from build123d import *

# Parameters (mm, degrees)
SKETCH1_R           = 57.5
SKETCH1_R_2         = 1.6
BOSS_EXTRUDE1_DEPTH = 10.6
FILLET1_R           = 2.5


with BuildPart() as part:
    # Sketch1 → Boss-Extrude1 (new body)
    with BuildSketch(Plane(origin=(0, 0, 0), x_dir=(1, 0, 0), z_dir=(0, 1, 0))):
        with Locations(Location((0, 0, 0), (0, 0, 270))):
            Circle(SKETCH1_R)
        with Locations(Location((-27, -46.765371804, 0), (0, 0, 270))):
            Circle(SKETCH1_R_2, mode=Mode.SUBTRACT)
        with Locations(Location((-46.765371804, -27, 0), (0, 0, 270))):
            Circle(SKETCH1_R_2, mode=Mode.SUBTRACT)
        with Locations(Location((-54, 0, 0), (0, 0, 270))):
            Circle(SKETCH1_R_2, mode=Mode.SUBTRACT)
        with Locations(Location((0, -54, 0), (0, 0, 270))):
            Circle(SKETCH1_R_2, mode=Mode.SUBTRACT)
        with Locations(Location((27, -46.765371804, 0), (0, 0, 270))):
            Circle(SKETCH1_R_2, mode=Mode.SUBTRACT)
        with BuildLine():
            ThreePointArc((43.742247125, 10.564838686), (44.135337618, 8.779064491), (44.455555556, 6.978795043))
            ThreePointArc((44.455555556, 6.978795043), (49.753361384, 5.138633627), (52, 0))
            ThreePointArc((52, 0), (49.753361384, -5.138633627), (44.455555556, -6.978795043))
            ThreePointArc((44.455555556, -6.978795043), (44.135337618, -8.779064491), (43.742247125, -10.564838686))
            ThreePointArc((43.742247125, -10.564838686), (47.23910353, -13.108193036), (48.574578963, -17.220754456))
            ThreePointArc((48.574578963, -17.220754456), (45.234108152, -23.187985482), (38.400908644, -23.459970489))
            ThreePointArc((38.400908644, -23.459970489), (37.416132554, -25.000660486), (36.369578094, -26.500071496))
            ThreePointArc((36.369578094, -26.500071496), (38.177808401, -28.89135937), (38.819805153, -31.819805153))
            ThreePointArc((38.819805153, -31.819805153), (34.244868492, -38.386316236), (26.500071496, -36.369578094))
            ThreePointArc((26.500071496, -36.369578094), (25.000660486, -37.416132554), (23.459970489, -38.400908644))
            ThreePointArc((23.459970489, -38.400908644), (24.027901885, -39.942787345), (24.220754456, -41.574578963))
            ThreePointArc((24.220754456, -41.574578963), (18.318158122, -48.488022764), (10.564838686, -43.742247125))
            ThreePointArc((10.564838686, -43.742247125), (8.779064491, -44.135337618), (6.978795043, -44.455555556))
            ThreePointArc((6.978795043, -44.455555556), (6.994696752, -44.727571384), (7, -45))
            ThreePointArc((7, -45), (-0.272428616, -51.994696752), (-6.978795043, -44.455555556))
            ThreePointArc((-6.978795043, -44.455555556), (-8.779064491, -44.135337618), (-10.564838686, -43.742247125))
            ThreePointArc((-10.564838686, -43.742247125), (-19.899538483, -48.041735691), (-23.459970489, -38.400908644))
            ThreePointArc((-23.459970489, -38.400908644), (-25.000660486, -37.416132554), (-26.500071496, -36.369578094))
            ThreePointArc((-26.500071496, -36.369578094), (-36.769552622, -36.769552622), (-36.369578094, -26.500071496))
            ThreePointArc((-36.369578094, -26.500071496), (-37.416132554, -25.000660486), (-38.400908644, -23.459970489))
            ThreePointArc((-38.400908644, -23.459970489), (-48.041735691, -19.899538483), (-43.742247125, -10.564838686))
            ThreePointArc((-43.742247125, -10.564838686), (-44.135337618, -8.779064491), (-44.455555556, -6.978795043))
            ThreePointArc((-44.455555556, -6.978795043), (-52, 0), (-44.455555556, 6.978795043))
            ThreePointArc((-44.455555556, 6.978795043), (-44.135337618, 8.779064491), (-43.742247125, 10.564838686))
            ThreePointArc((-43.742247125, 10.564838686), (-48.041735691, 19.899538483), (-38.400908644, 23.459970489))
            ThreePointArc((-38.400908644, 23.459970489), (-37.416132554, 25.000660486), (-36.369578094, 26.500071496))
            ThreePointArc((-36.369578094, 26.500071496), (-36.769552622, 36.769552622), (-26.500071496, 36.369578094))
            ThreePointArc((-26.500071496, 36.369578094), (-25.000660486, 37.416132554), (-23.459970489, 38.400908644))
            ThreePointArc((-23.459970489, 38.400908644), (-19.899538483, 48.041735691), (-10.564838686, 43.742247125))
            ThreePointArc((-10.564838686, 43.742247125), (-8.779064491, 44.135337618), (-6.978795043, 44.455555556))
            ThreePointArc((-6.978795043, 44.455555556), (-0.272428616, 51.994696752), (7, 45))
            ThreePointArc((7, 45), (6.994696752, 44.727571384), (6.978795043, 44.455555556))
            ThreePointArc((6.978795043, 44.455555556), (8.779064491, 44.135337618), (10.564838686, 43.742247125))
            ThreePointArc((10.564838686, 43.742247125), (18.318158122, 48.488022764), (24.220754456, 41.574578963))
            ThreePointArc((24.220754456, 41.574578963), (24.027901885, 39.942787345), (23.459970489, 38.400908644))
            ThreePointArc((23.459970489, 38.400908644), (25.000660486, 37.416132554), (26.500071496, 36.369578094))
            ThreePointArc((26.500071496, 36.369578094), (34.244868492, 38.386316236), (38.819805153, 31.819805153))
            ThreePointArc((38.819805153, 31.819805153), (38.177808401, 28.89135937), (36.369578094, 26.500071496))
            ThreePointArc((36.369578094, 26.500071496), (37.416132554, 25.000660486), (38.400908644, 23.459970489))
            ThreePointArc((38.400908644, 23.459970489), (45.234108152, 23.187985482), (48.574578963, 17.220754456))
            ThreePointArc((48.574578963, 17.220754456), (47.23910353, 13.108193036), (43.742247125, 10.564838686))
        make_face(mode=Mode.SUBTRACT)
        with Locations(Location((46.765371804, -27, 0), (0, 0, 270))):
            Circle(SKETCH1_R_2, mode=Mode.SUBTRACT)
        with Locations(Location((-46.765371804, 27, 0), (0, 0, 270))):
            Circle(SKETCH1_R_2, mode=Mode.SUBTRACT)
        with Locations(Location((-27, 46.765371804, 0), (0, 0, 270))):
            Circle(SKETCH1_R_2, mode=Mode.SUBTRACT)
        with Locations(Location((54, 0, 0), (0, 0, 270))):
            Circle(SKETCH1_R_2, mode=Mode.SUBTRACT)
        with Locations(Location((46.765371804, 27, 0), (0, 0, 270))):
            Circle(SKETCH1_R_2, mode=Mode.SUBTRACT)
        with Locations(Location((0, 54, 0), (0, 0, 270))):
            Circle(SKETCH1_R_2, mode=Mode.SUBTRACT)
        with Locations(Location((27, 46.765371804, 0), (0, 0, 270))):
            Circle(SKETCH1_R_2, mode=Mode.SUBTRACT)
    extrude(amount=BOSS_EXTRUDE1_DEPTH)

    # Fillet1
    # the kernel refuses this fillet: 2.5 mm, written as the material it takes off along each edge
    with BuildSketch(Plane(origin=(43.742247125, -4.820377086, -10.564838686), x_dir=(0.21389520927514544, 0, 0.9768566115091517), z_dir=(0, 1, 0)), Plane(origin=(44.455555556, -4.820377086, 6.978795043), x_dir=(-0.17621343506931061, 0, 0.9843519824234996), z_dir=(0, 1, 0)), Plane(origin=(38.400908644, -4.820377086, 23.459970489), x_dir=(-0.5394951813032318, 0, 0.841988687186825), z_dir=(0, 1, 0)), Plane(origin=(26.500071496, -4.820377086, 36.369578094), x_dir=(-0.8206436767197667, 0, 0.5714402469723874), z_dir=(0, 1, 0)), Plane(origin=(10.564838686, -4.820377086, 43.742247125), x_dir=(-0.9768566115091482, 0, 0.21389520927516179), z_dir=(0, 1, 0)), Plane(origin=(-6.978795043, -4.820377086, 44.455555556), x_dir=(-0.9843519824235082, 0, -0.1762134350692629), z_dir=(0, 1, 0)), Plane(origin=(-23.459970489, -4.820377086, 38.400908644), x_dir=(-0.8419886871868016, 0, -0.5394951813032682), z_dir=(0, 1, 0)), Plane(origin=(-36.369578094, -4.820377086, 26.500071496), x_dir=(-0.5714402469723492, 0, -0.8206436767197933), z_dir=(0, 1, 0)), Plane(origin=(23.459970489, -4.820377086, -38.400908644), x_dir=(0.8419886871867822, 0, 0.5394951813032985), z_dir=(0, 1, 0)), Plane(origin=(6.978795043, -4.820377086, -44.455555556), x_dir=(0.9843519824234905, 0, 0.1762134350693622), z_dir=(0, 1, 0)), Plane(origin=(-10.564838686, -4.820377086, -43.742247125), x_dir=(0.9768566115091611, 0, -0.21389520927510192), z_dir=(0, 1, 0)), Plane(origin=(-26.500071496, -4.820377086, -36.369578094), x_dir=(0.8206436767197971, 0, -0.5714402469723435), z_dir=(0, 1, 0)), Plane(origin=(-38.400908644, -4.820377086, -23.459970489), x_dir=(0.5394951813033058, 0, -0.8419886871867777), z_dir=(0, 1, 0)), Plane(origin=(-44.455555556, -4.820377086, -6.978795043), x_dir=(0.17621343506938397, 0, -0.9843519824234865), z_dir=(0, 1, 0)), Plane(origin=(-43.742247125, -4.820377086, 10.564838686), x_dir=(-0.21389520927510172, 0, -0.9768566115091614), z_dir=(0, 1, 0))) as fillet1_piece_1:
        with BuildLine():
            CenterArc((1.98171058, 2.499426205), FILLET1_R, 199.641418976, 69.130988159)
            ThreePointArc((-0.372826194, 1.659094972), (-0.135846618, 0.840910614), (0, 0))
            ThreePointArc((0, 0), (0.964075417, 0.010328312), (1.928150834, 0))
        make_face()
    extrude(amount=20.240754172, mode=Mode.SUBTRACT)
    with BuildSketch(Plane(origin=(38.400908644, -4.820377086, -23.459970489), x_dir=(0.9397859916311062, 0, -0.34176350000247), z_dir=(0, 1, 0)), Plane(origin=(26.500071496, -4.820377086, -36.369578094), x_dir=(0.7374618133707781, 0, -0.6753888315776947), z_dir=(0, 1, 0)), Plane(origin=(44.455555556, -4.820377086, -6.978795043), x_dir=(0.9990362718468525, 0, 0.043892226354353435), z_dir=(0, 1, 0)), Plane(origin=(43.742247125, -4.820377086, 10.564838686), x_dir=(0.9061923359602189, 0, 0.42286575913280305), z_dir=(0, 1, 0)), Plane(origin=(36.369578094, -4.820377086, 26.500071496), x_dir=(0.6753888315777279, 0, 0.7374618133707476), z_dir=(0, 1, 0)), Plane(origin=(23.459970489, -4.820377086, 38.400908644), x_dir=(0.3417635000024204, 0, 0.9397859916311243), z_dir=(0, 1, 0)), Plane(origin=(6.978795043, -4.820377086, 44.455555556), x_dir=(-0.043892226354455326, 0, 0.9990362718468481), z_dir=(0, 1, 0)), Plane(origin=(-10.564838686, -4.820377086, 43.742247125), x_dir=(-0.4228657591328737, 0, 0.9061923359601859), z_dir=(0, 1, 0)), Plane(origin=(-26.500071496, -4.820377086, 36.369578094), x_dir=(-0.7374618133709434, 0, 0.6753888315775142), z_dir=(0, 1, 0)), Plane(origin=(10.564838686, -4.820377086, -43.742247125), x_dir=(0.4228657591329353, 0, -0.9061923359601571), z_dir=(0, 1, 0)), Plane(origin=(-6.978795043, -4.820377086, -44.455555556), x_dir=(0.04389222635458482, 0, -0.9990362718468423), z_dir=(0, 1, 0)), Plane(origin=(-23.459970489, -4.820377086, -38.400908644), x_dir=(-0.3417635000022023, 0, -0.9397859916312036), z_dir=(0, 1, 0)), Plane(origin=(-36.369578094, -4.820377086, -26.500071496), x_dir=(-0.6753888315774389, 0, -0.7374618133710125), z_dir=(0, 1, 0)), Plane(origin=(-43.742247125, -4.820377086, -10.564838686), x_dir=(-0.9061923359601008, 0, -0.422865759133056), z_dir=(0, 1, 0)), Plane(origin=(-44.455555556, -4.820377086, 6.978795043), x_dir=(-0.9990362718468366, 0, -0.04389222635471359), z_dir=(0, 1, 0)), Plane(origin=(-38.400908644, -4.820377086, 23.459970489), x_dir=(-0.9397859916312232, 0, 0.3417635000021483), z_dir=(0, 1, 0))) as fillet1_piece_2:
        with BuildLine():
            CenterArc((2.004124414, 2.481490179), FILLET1_R, 193.892520635, 69.130988159)
            ThreePointArc((-0.422745168, 1.881236871), (-0.201295571, 0.942882908), (0, 0))
            ThreePointArc((0, 0), (0.8502346, 0.051827497), (1.700469199, 0))
        make_face()
    extrude(amount=20.240754172, mode=Mode.SUBTRACT)
    with BuildSketch(Plane(origin=(36.369578094, -4.820377086, -26.500071496), x_dir=(0.6753888315776805, 0, -0.7374618133707912), z_dir=(0, 1, 0))) as fillet1_piece_3:
        with BuildLine():
            CenterArc((2.004124414, -2.481490179), FILLET1_R, 96.976491207, 69.130988159)
            ThreePointArc((-0.422745168, -1.881236871), (-0.201295571, -0.942882908), (0, 0))
            ThreePointArc((0, 0), (0.8502346, -0.051827497), (1.700469199, 0))
        make_face()
    extrude(amount=20.240754172, mode=Mode.SUBTRACT)


solid = part.part
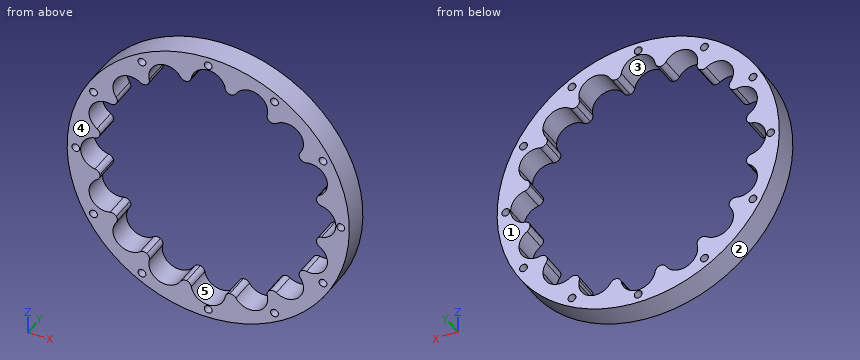
CAD build for the part. Positions are in the model's coordinates, mm. Face numbers are marked on the shaded views. A direction names the side the tool comes from. Give positions to 0.01 mm unless a question says otherwise; leave off trailing zeros. Order: outer loops, then holes, each group sorted by start corner. A loop starts at its lowest first (then second) coordinate and runs counter-clockwise, first axis right, second up. Notation, with made-up numbers: (32, 35.5) -> (41, 35.5) arc R19 ccw to (41, 40.5) -> close; hole circle Ø9 at (61.25, 72). An arc over 180 degrees is marked (long way). Return JSON: item names as keys, results as strings.
Q1. Drill centre lines: line 1 (X direction, y = 7, z = 0); line 2 (X direction, y = 9.25, z = -47); line 3 (X direction, y = 8, z = -28). Where is each one in solid material? Low to high.
Working result:
{"line 1": "-57.5 to -55.6, -52.4 to -52, 52 to 52.4, 55.6 to 57.5", "line 2": "-33.12 to -28.58, -25.42 to -21.64, -12.8 to -6.71, 6.71 to 12.8, 21.64 to 25.42, 28.58 to 33.12", "line 3": "-50.22 to -48.01, -45.52 to -37.69, 37.69 to 45.52, 48.01 to 50.22"}
Q2. Saw through at A-A (x = 0). Write the cut outline in (y, z), then the cut area to 3 significant figures.
Working result:
{"outline": "(0, -57.5) -> (10.6, -57.5) -> (10.6, -55.6) -> (0, -55.6) -> close; (0, -52.4) -> (10.6, -52.4) -> (10.6, -52) -> (0, -52) -> close; (0, 52) -> (10.6, 52) -> (10.6, 52.4) -> (0, 52.4) -> close; (0, 55.6) -> (10.6, 55.6) -> (10.6, 57.5) -> (0, 57.5) -> close", "area": "48.8 mm²"}
Q3. Which spindle directions (+Z, -Z, +X, -X, +Y, -Y) get a long thin tool onto all of the face, cutting with end or side? Do the marked faces 4 and 5. Say none if no direction does.
Working result:
{"face 4": "+Z, -Z, +X, -X, -Y", "face 5": "+Y, -Y"}
Q4. Flat gauge pins, fed straight in: pin 1 (6 mm diameter, centred on x = 31.5, y = 8.5, fed in from +Z); pin 2 (4 mm diameter, centred on x = 46.77, z = -27, fed in from +Y); pin 3 (2 mm diameter, centred on y = 4, z = 23.5, fed in from -X) (3 decimals); pin 4 (6 mm diameter, centred on y = 6, z = -0.5, fed in from +X). Where does each tip first touch, or does it go through?
Working result:
{"pin 1": "z = 49.94", "pin 2": "y = 10.6", "pin 3": "x = -52.915", "pin 4": "x = 57.5"}
Q5. Mould opens along Z. For the marked faces 1, 2 and 3 say: pulls with the +Z half, pulls with the -Z half, needs draft (parallel to the pull), parting line crosses it, or undercut.
Working result:
{"face 1": "needs draft", "face 2": "parting line crosses it", "face 3": "undercut"}
Q6. Saw through at D-D (y = 3). Count the separate pieces of the cut face and the enclosed holes in it, then the cut area to 3 significant figures.
Working result:
{"separate pieces": "1", "enclosed holes": "13", "area": "2,630 mm²"}
Q7. Saw through at B-B (x = -16). Write the cut outline in (y, z).
Working result:
{"outline": "(0, -55.23) -> (10.6, -55.23) -> (10.6, -48.47) -> (0, -48.47) -> close; (0, 48.47) -> (10.6, 48.47) -> (10.6, 55.23) -> (0, 55.23) -> close"}
Q8. Saw through at C-C (z = -15). Write the cut outline in (x, y), then the cut area to 3 significant figures.
Working result:
{"outline": "(-55.51, 0) -> (-48.21, 0) -> (-48.21, 10.6) -> (-55.51, 10.6) -> close; (48.21, 0) -> (55.51, 0) -> (55.51, 10.6) -> (48.21, 10.6) -> close", "area": "155 mm²"}
